Verification items for the finished model (mm, model axes). Face numbers are marked on the shaded views. A direction names the side the tool comes from. Round coordinates to 2 decimals unless told otherwise and drop trailing zeros. Order: outer loops, then holes, each group sorted by start corner. A loop starts at its lowest first (then second) coordinate and runs counter-clockwise, first axis right, second up. Notation, with made-up numbers: M 20.25,-16 L 25.25,-16 A8 cw 25.25,-12 Z; hole C 82.5,75.25 d5. An arc over 180 degrees is marked long. Use CSV: the item, a comma, the result in double quotes. Start each with the question number.
Q1. Sectioned sample at D-D (z = -5). Enter the section's corners in (x, y).
Q2. Sectioned sample at C-C (x = 4.5). Enter the section's corners in (y, z), and give its area (4 significant figures).
Q3. Scan lines: line 1 (Y direction, x = 1.2, z = -10); line 2 (Z direction, x = 7.75, y = 45.5); line 3 (X direction, y = 3.5, z = -12). Record each from-to range of solid material in increasing order.
Q4. Gauge pin test, flat end, axial feed: pin 1 Ø2 at (x, z) = (3.5, -10) entering from -Y. Record the tip position at first contact, or that the pin passes through.
Q5. Sectioned sample at B-B (z = -10). Enter the section's corners in (x, y), and give its area (3 significant figures).
Q6. Sectioned sample at A-A (y = 12.5). Enter the section's corners in (x, z), and give its area (3 significant figures).
Q7. Mould release check, pull along X, two halves, no side actions. Record for the marked faces 1, 2 and 3: +X half, -X half, draft (parallel to the pull), parting line (faces both ways), or undercut.
Q8. Set-up check for the marked faces 4 and 5: record each of +Z, -Z, +X, -X, +Y, -Y from which the full face is reachable in a straight line by a thin tool's end or side.
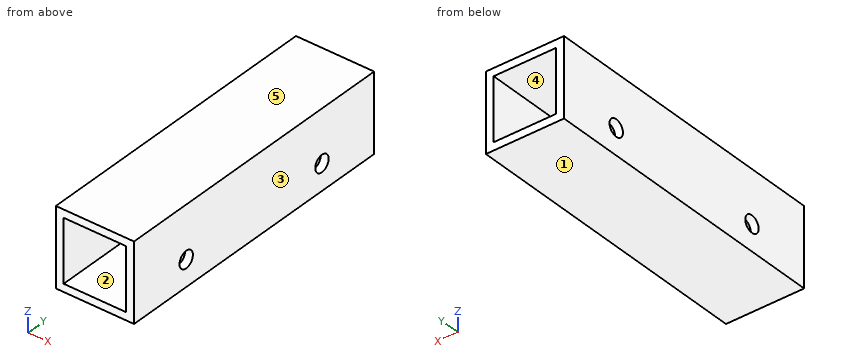
```python
from build123d import *

# Parameters (mm, degrees)
SKETCH_1_W              = 15
SKETCH_1_H              = 15
SKETCH_1_W_2            = 12
SKETCH_1_H_2            = 12
EXTRUDE_1_DEPTH         = 57.5
CUT_EXTRUDE_1_OUTLINE_R = 1.6
CUT_EXTRUDE_1_DEPTH     = 15


# Read off the part's stored shape, not the designer's step: 切除-拉伸1
with BuildPart() as part:
    # 草图1 → 凸台-拉伸1 (new body)
    with BuildSketch(Plane(origin=(0, 0, 0), x_dir=(1, 0, 0), z_dir=(0, 1, 0))):
        with Locations((7.5, 7.5)):
            Rectangle(SKETCH_1_W, SKETCH_1_H)
        with Locations((7.5, 7.5)):
            Rectangle(SKETCH_1_W_2, SKETCH_1_H_2, mode=Mode.SUBTRACT)
    extrude(amount=EXTRUDE_1_DEPTH)

    # 切除-拉伸1 outline → 切除-拉伸1 (cut)
    with BuildSketch(Plane.YZ):
        with Locations((45, -10)):
            Circle(CUT_EXTRUDE_1_OUTLINE_R)
        with Locations((12.5, -10)):
            Circle(CUT_EXTRUDE_1_OUTLINE_R)
    extrude(amount=CUT_EXTRUDE_1_DEPTH, mode=Mode.SUBTRACT)


solid = part.part
```
Verdict:
1,outline,"M 0,0 L 1.5,0 L 1.5,57.5 L 0,57.5 Z; M 13.5,0 L 15,0 L 15,57.5 L 13.5,57.5 Z"
2,outline,"M 0,-15 L 57.5,-15 L 57.5,-13.5 L 0,-13.5 Z; M 0,-1.5 L 57.5,-1.5 L 57.5,0 L 0,0 Z"
2,area,"172.5 mm²"
3,line 1,"y = 0 to 10.9, 14.1 to 43.4, 46.6 to 57.5"
3,line 2,"z = -15 to -13.5, -1.5 to 0"
3,line 3,"x = 0 to 1.5, 13.5 to 15"
4,pin 1,"passes through"
5,outline,"M 0,0 L 1.5,0 L 1.5,10.9 L 0,10.9 Z; M 0,14.1 L 1.5,14.1 L 1.5,43.4 L 0,43.4 Z; M 0,46.6 L 1.5,46.6 L 1.5,57.5 L 0,57.5 Z; M 13.5,0 L 15,0 L 15,10.9 L 13.5,10.9 Z; M 13.5,14.1 L 15,14.1 L 15,43.4 L 13.5,43.4 Z; M 13.5,46.6 L 15,46.6 L 15,57.5 L 13.5,57.5 Z"
5,area,"153 mm²"
6,outline,"M 0,-15 L 15,-15 L 15,-11.6 L 13.5,-11.6 L 13.5,-13.5 L 1.5,-13.5 L 1.5,-11.6 L 0,-11.6 Z; M 0,-8.4 L 1.5,-8.4 L 1.5,-1.5 L 13.5,-1.5 L 13.5,-8.4 L 15,-8.4 L 15,0 L 0,0 Z"
6,area,"71.4 mm²"
7,face 1,"draft"
7,face 2,"undercut"
7,face 3,"+X half"
8,face 4,"+Y, -Y"
8,face 5,"+Z, +X, -X, +Y, -Y"
